Input: dimensioned drawing with shaded views. Units: mm. Origin: part minimum x, y, z. Give positions to 0.01 mm unless a question says otherwise; leave off trailing zeros. Loops run counter-clockwise (first coordinate to the right, second up) from the corner with the lowest first, then second, coordinate; pieces in that order, holes last. Notation, with made-up numbers: (-36, 79.25) -> (22, 79.25) arc R27 cw to (22, 105.25) -> close; hole circle Ø4 at (26.5, 36). An arc over 180 degrees is marked (long way). One line per question, with ' | ' between items. Start each with the question number.
Item 1: Section D-D on x = 81.5. Return loops of the section in (y, z) (1 decimal).
Item 2: Pin query (flat end, axial travel): P1, Ø5.5, axis at x = 92.202, y = 6.35, coming from the -Z side; P2, Ø2, axis at y = 19, z = 3.5, coming from the +X side (1 decimal); P3, Ø1, axis at y = 3.5, z = 10, coming from the +X side; P4, Ø2, axis at y = 18.5, z = 3.5, coming from the +X side. Return the tip coordinate at first contact, or that it passes through.
Item 3: Material intervals for line 1 along Y through (x, z) = (64, 10.25) (1 decimal); line 2 along Y through (x, z) = (89.5, 4.75) (1 decimal); line 3 along X through (y, z) = (11.5, 3.5) (1 decimal), sorted ascending. Write a range as [from, to].
Item 4: Mould query, pull axis Y, two halves, no side actions, for the marked faces 1, 2, 3 and 4. Classes: released by +Y, released by -Y, zero draft, split by the parting line, or undercut.
Item 5: Section C-C on z = 15. Give the number of separate pieces and of enclosed holes in the cut face, then the cut area to 3 significant figures.
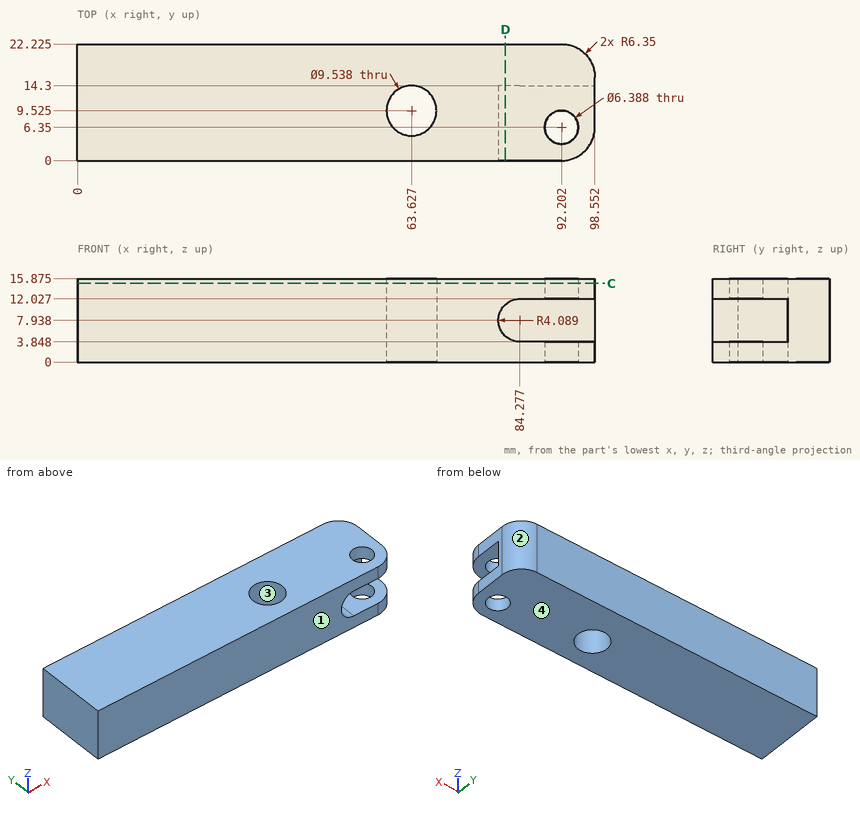
Result sheet:
1) outline: (0, 0) -> (22.2, 0) -> (22.2, 15.9) -> (0, 15.9) -> (0, 10.9) -> (14.3, 10.9) -> (14.3, 4.9) -> (0, 4.9) -> close
2) P1: passes through | P2: stops at x = 98.2 | P3: stops at x = 81.09 | P4: stops at x = 98.34
3) line 1: y = [0, 4.8], [14.3, 22.2] | line 2: y = [14.3, 22.2] | line 3: x = [0, 59.3], [68, 98.6]
4) face 1: released by -Y | face 2: released by +Y | face 3: undercut | face 4: zero draft
5) separate pieces: 1 | enclosed holes: 2 | area: 2,070 mm²
